Geometry: final body of the model. Coordinates: model frame, mm. Face numbers are marked on the shaded views. A direction names the side the tool comes from. Give positions to 0.01 mm unless a question says otherwise; leave off trailing zeros. Write each loop counter-clockwise with the first axis right and the second up, starting at its lowest first coordinate (ties: lowest second). Pieces come first, ordered by that corner, then holes.
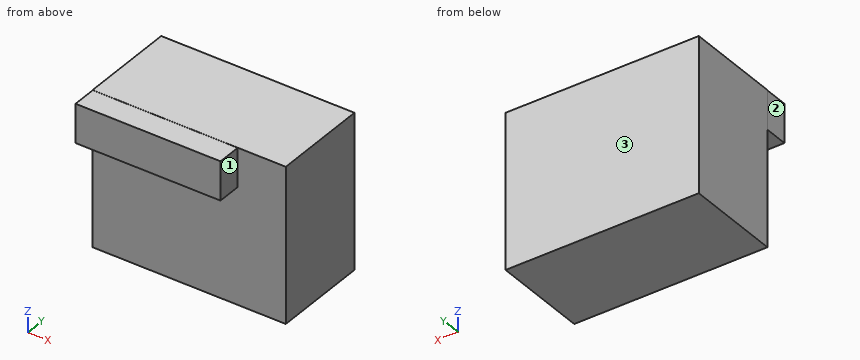
from build123d import *

# Parameters (mm, degrees)
F0_W     = 101.6
F0_H     = 50.8
F1_DEPTH = 81.28
F3_W     = 76.2
F3_H     = 20.32
F4_DEPTH = 12.7


with BuildPart() as f1:
    # F0 (on Top) → F1 (new body)
    with BuildSketch(Plane.XY):
        Rectangle(F0_W, F0_H)
    extrude(amount=F1_DEPTH)

    # F3 (on offset) → F4 (join)
    with BuildSketch(Plane.XZ.offset(25.4)):
        with Locations((-12.610486, 71.049867)):
            Rectangle(F3_W, F3_H)
    extrude(amount=F4_DEPTH)


solid = f1.part
Q1. Ray query, line 1 along Y through (x, z) = (-8, 34). Return the intervals inside material, ascending.
Filled sheet:
line 1: y = -25.4 to 25.4
Q2. Access query for the marked faces 1, 2 and 3. Directions: +Z, -Z, +X, -X, +Y, -Y. A direction counts if a zero-diameter tool reaches every point of the face in a straight line with its end or side. Return the directions, or none.
Filled sheet:
face 1: +Z, -Z, +X, -Y
face 2: +Z, -Z, -X, -Y
face 3: +Z, -Z, +X, -X, +Y
Q3. Section C-C on y = -30.5. Output: boundary loops of the cut face in (x, z), plus the area to 3 significant figures.
Filled sheet:
outline: (-50.71, 60.89) - (25.49, 60.89) - (25.49, 81.21) - (-50.71, 81.21) - close
area: 1,550 mm2
Q4. Section B-B on z = 28. Output: boundary loops of the cut face in (x, y), plus the area to 3 significant figures.
Filled sheet:
outline: (-50.8, -25.4) - (50.8, -25.4) - (50.8, 25.4) - (-50.8, 25.4) - close
area: 5,160 mm2
Q5. Section A-A on x = 22. Output: boundary loops of the cut face in (y, z).
Filled sheet:
outline: (-38.1, 60.89) - (-25.4, 60.89) - (-25.4, 0) - (25.4, 0) - (25.4, 81.28) - (-25.4, 81.28) - (-25.4, 81.21) - (-38.1, 81.21) - close
Q6. Pin query (flat end, axial travel): P1, Ø10, axis at x = 1.5, y = -35, coming from the -Z side; P2, Ø4, axis at y = -32.5, z = 68, coming from the -X side; P3, Ø14, axis at y = -34, z = 74, coming from the +X side. Return the tip coordinate at first contact, or that it passes through.
Filled sheet:
P1: stops at z = 60.89
P2: stops at x = -50.71
P3: stops at x = 25.49
